The model under review builds one solid part; all positions refer to its coordinate system, in mm. A direction names the side the tool comes from. Give positions to 0.01 mm unless a question says otherwise; leave off trailing zeros. Write each question's results on one line, items separated by ' | '. Start each with the question number.
from build123d import *

# Parameters (mm, degrees)
CROQUIS1_W              = 100
CROQUIS1_H              = 84
SALIENTE_EXTRUIR1_DEPTH = 5
CROQUIS2_W              = 89
CROQUIS2_H              = 75
SALIENTE_EXTRUIR2_DEPTH = 19
SALIENTE_EXTRUIR2_TAPER = 6
CROQUIS3_R              = 2.25
SALIENTE_EXTRUIR3_DEPTH = 49.5


with BuildPart() as part:
    # Croquis1 → Saliente-Extruir1 (new body)
    with BuildSketch(Plane.XY):
        Rectangle(CROQUIS1_W, CROQUIS1_H)
    extrude(amount=SALIENTE_EXTRUIR1_DEPTH)

    # Croquis2 → Saliente-Extruir2 (add)
    with BuildSketch(Plane(origin=(0, 0, 0), x_dir=(-1, 0, 0), z_dir=(0, 0, -1))):
        Rectangle(CROQUIS2_W, CROQUIS2_H)
    extrude(amount=SALIENTE_EXTRUIR2_DEPTH, taper=SALIENTE_EXTRUIR2_TAPER)

    # Croquis3 → Saliente-Extruir3 (add, symmetric)
    with BuildSketch(Plane(origin=(0, 0, 0), x_dir=(0, 0, -1), z_dir=(1, 0, 0))):
        with BuildLine():
            Line((0, 12), (10.1, 12))
            ThreePointArc((10.1, 12), (14.271930009, 10.271930009), (16, 6.1))
            Line((16, 6.1), (16, 5.9))
            ThreePointArc((16, 5.9), (14.271930009, 1.728069991), (10.1, 0))
            Line((10.1, 0), (0, 0))
            Line((0, 0), (0, 12))
        make_face()
        with Locations(Location((10.1, 5.9, 0), (0, 0, 180))):
            Circle(CROQUIS3_R, mode=Mode.SUBTRACT)
    extrude(amount=SALIENTE_EXTRUIR3_DEPTH, both=True)


solid = part.part
(1) Wall thickness on L1, parallel to Y at x = 47, z = -10.1; L2, parallel to Z at x = -47.25, y = 5.9; L3, parallel to Z at x = -46, y = 5: over which ranges is each line inside the solid? List them lowest first.
(2) Machinability: for faces 1 (the flat face through (47, 0, -5)), 2 (the cylindrical face through (-46.112, 10.318, -14.226)), 3 (the flat face through (47, 12, -5)), 4 (the flat face through (-49.5, 6, -6)), 5 (the flat face through (49.5, 6, -6)), which of the approach directions +Z, -Z, +X, -X, +Y, -Y give a long, thin tool a straight path to every point of the face, cutting with its end or side? Answer none if there is none.
(3) Clearance check with flat-ended pins moving along their axes: P1, Ø5, axis at x = -46.5, z = -4, coming from the +Y side; P2, Ø1.8, axis at x = -46, z = -4.5, coming from the -Y side; P3, Ø3, axis at x = 46, z = -3, coming from the +Y side. State where each tip first meets the part, or that it passes through.
(4) Draft analysis for pull direction Z (two halves, no side actions). For faces 6 (the flat face through (-46, 0, -5)), 7 (the cylindrical face through (46.307, 5.801, -12.348)), 8 (the flat face through (-1, 1, 5)), state which applies: pulls with the +Z half, pulls with the -Z half, needs draft (parallel to the pull), parting line crosses it, or undercut.
Calculated:
1) L1: y = 0 to 3.65, 8.15 to 12 | L2: z = -16 to -12.35, -7.85 to 5 | L3: z = -15.93 to -12.16, -8.04 to 5
2) face 1: -Z, +X, -Y | face 2: -Z, -X, +Y | face 3: -Z, +X, +Y | face 4: -Z, -X, +Y, -Y | face 5: -Z, +X, +Y, -Y
3) P1: stops at y = 37.18 | P2: stops at y = 0 | P3: stops at y = 12
4) face 6: needs draft | face 7: undercut | face 8: pulls with the +Z half
